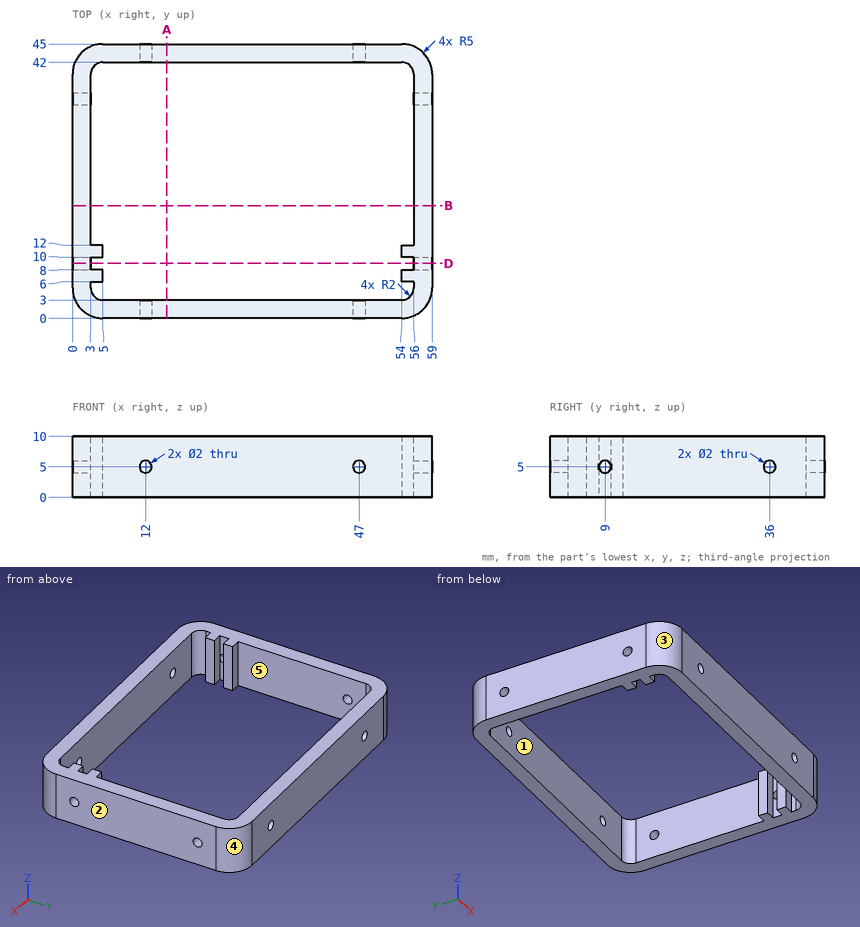
Drawing for the job (mm, zero at the part's lowest x, y, z). A direction names the side the tool comes from. Give positions to 0.01 mm unless a question says otherwise; leave off trailing zeros. Order: outer loops, then holes, each group sorted by start corner. A loop starts at its lowest first (then second) coordinate and runs counter-clockwise, first axis right, second up. Notation, with made-up numbers: (77.25, -14.75) -> (122.25, -14.75) arc R21 cw to (122.25, 2.25) -> close; hole circle Ø2 at (63.5, 38). An arc over 180 degrees is marked (long way). Use one line per item in the form item = value.
(1) Flat gauge pins, fed straight in: P1, Ø1.8, axis at y = 9, z = 5, coming from the -X side; P2, Ø1, axis at x = 3.5, z = 5, coming from the -Y side; P3, Ø1.6, axis at x = 4, z = 5.5, coming from the +Y side; P4, Ø1.6, axis at x = 4, z = 5.5, coming from the -Y side. Where does each tip first touch, or does it go through?
Solution:
P1 = through
P2 = 0.1
P3 = 45
P4 = 0
(2) Saw through at A-A (x = 15.5). Write the cut outline in (y, z).
Solution:
outline = (0, 0) -> (3, 0) -> (3, 10) -> (0, 10) -> close; (42, 0) -> (45, 0) -> (45, 10) -> (42, 10) -> close
(3) Drill centre lines: line 1 (Z direction, x = 12, y = 43.6); line 2 (X direction, y = 32, z = 2); line 3 (X direction, y = 1.5, z = 5). Where is each one in solid material? Low to high. Write a range as from..to.
Solution:
line_1 = 0..4, 6..10
line_2 = 0..3, 56..59
line_3 = 1.43..11, 13..46, 48..57.57
(4) Tool access for the marked faces 1 and 2: list every direction of +Z, -Z, +X, -X, +Y, -Y with a clear straight run to the whole face (end or side of a thin tool).
Solution:
face_1 = +Z, -Z
face_2 = +Z, -Z, +X, +Y, -Y
(5) Saw through at B-B (y = 18.5). Write the cut outline in (x, z), then the cut area to 3 significant figures.
Solution:
outline = (0, 0) -> (3, 0) -> (3, 10) -> (0, 10) -> close; (56, 0) -> (59, 0) -> (59, 10) -> (56, 10) -> close
area = 60.0 mm²
(6) Pull direction Y, two halves, no side cores. Call the marked faces 3, 4 and 5: +Y half, -Y half, draft (parallel to the pull), parting line (faces both ways), or undercut.
Solution:
face_3 = -Y half
face_4 = +Y half
face_5 = undercut
(7) Saw through at D-D (y = 9). Write the cut outline in (x, z).
Solution:
outline = (0, 0) -> (3, 0) -> (3, 4) -> (0, 4) -> close; (0, 6) -> (3, 6) -> (3, 10) -> (0, 10) -> close; (56, 0) -> (59, 0) -> (59, 4) -> (56, 4) -> close; (56, 6) -> (59, 6) -> (59, 10) -> (56, 10) -> close
